Build history of the part. All positions in model axes, mm. Give positions to 0.01 mm unless a question says otherwise; leave off trailing zeros. Loops run counter-clockwise (first coordinate to the right, second up) from the corner with the lowest first, then second, coordinate; pieces in that order, holes last. Notation, with made-up numbers: (0.25, 72) -> (34.25, 72) arc R33 ccw to (34.25, 105) -> close; hole circle Ø2 at (49.25, 57). An arc over 180 degrees is marked (long way). Answer as a JSON object with one key per item and string values. Group by question number.
Q1. Band-saw the part on D-D, the plane x = 14.5. Write the cut outline in (y, z).
Q2. Wall check: probe 1 along Z at (x, y) = (1.5, 0.1); probe 2 along Z at (x, y) = (1, 0.8); probe 3 along X at (y, z) = (0.35, -5.9). Give the ranges that are in metal, low to high. Write a range as from..to.
Q3. Band-saw the part on B-B, the plane x = 1.6. Write the cut outline in (y, z), plus the area to 3 significant figures.
Q4. Band-saw the part on C-C, the plane y = 0.2. Write the cut outline in (x, z), plus the area to 3 significant figures.
Q5. Band-saw the part on A-A, the plane z = 5.9. Write the cut outline in (x, y), plus the area to 3 significant figures.
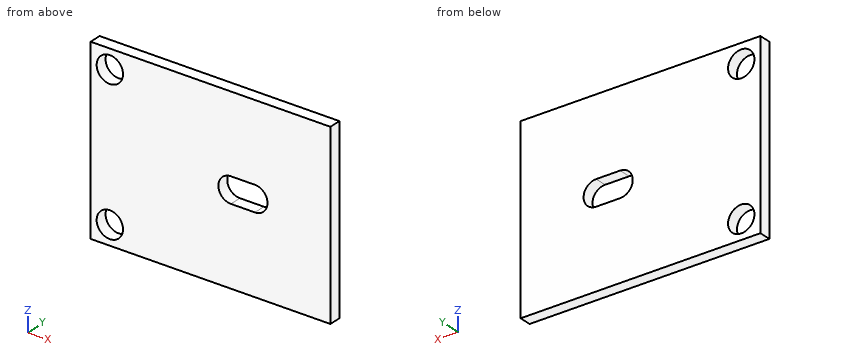
from build123d import *

# Parameters (mm, degrees)
ESQUISSE1_W             = 20
ESQUISSE1_H             = 15
BOSS_EXTRU_1_DEPTH      = 1
ESQUISSE2_R             = 1.1
ENL_V_MAT_EXTRU_1_DEPTH = 22.38340478


with BuildPart() as part:
    # Esquisse1 → Boss.-Extru.1 (new body)
    with BuildSketch(Plane(origin=(0, 0, 0), x_dir=(1, 0, 0), z_dir=(0, 1, 0))):
        with Locations((10, 0)):
            Rectangle(ESQUISSE1_W, ESQUISSE1_H)
    extrude(amount=BOSS_EXTRU_1_DEPTH)

    # Esquisse2 → Enlèv. mat.-Extru.1 (cut, through all)
    with BuildSketch(Plane(origin=(0, 1, 0), x_dir=(1, 0, 0), z_dir=(0, 1, 0))):
        with Locations(Location((1.6, 5.9, 0), (0, 0, 270))):
            Circle(ESQUISSE2_R)
        with Locations(Location((1.6, -5.9, 0), (0, 0, 270))):
            Circle(ESQUISSE2_R)
        with BuildLine():
            Line((11.7, 1.05), (13.7, 1.05))
            ThreePointArc((13.7, 1.05), (14.75, 0), (13.7, -1.05))
            Line((13.7, -1.05), (11.7, -1.05))
            ThreePointArc((11.7, -1.05), (10.65, 0), (11.7, 1.05))
        make_face()
    extrude(amount=-ENL_V_MAT_EXTRU_1_DEPTH, mode=Mode.SUBTRACT)


solid = part.part
Worked answers:
{
 "1": {"outline": "(0, -7.5) -> (1, -7.5) -> (1, -0.68) -> (0, -0.68) -> close; (0, 0.68) -> (1, 0.68) -> (1, 7.5) -> (0, 7.5) -> close"},
 "2": {"probe 1": "-7.5..-7, -4.8..4.8, 7..7.5", "probe 2": "-7.5..-6.82, -4.98..4.98, 6.82..7.5", "probe 3": "0..0.5, 2.7..20"},
 "3": {"outline": "(0, -7.5) -> (1, -7.5) -> (1, -7) -> (0, -7) -> close; (0, -4.8) -> (1, -4.8) -> (1, 4.8) -> (0, 4.8) -> close; (0, 7) -> (1, 7) -> (1, 7.5) -> (0, 7.5) -> close", "area": "10.6 mm2"},
 "4": {"outline": "(0, -7.5) -> (20, -7.5) -> (20, 7.5) -> (0, 7.5) -> close; hole circle Ø2.2 at (1.6, -5.9); hole circle Ø2.2 at (1.6, 5.9); hole (11.7, -1.05) -> (13.7, -1.05) arc R1.05 ccw to (13.7, 1.05) -> (11.7, 1.05) arc R1.05 ccw to start", "area": "285 mm2"},
 "5": {"outline": "(0, 0) -> (0.5, 0) -> (0.5, 1) -> (0, 1) -> close; (2.7, 0) -> (20, 0) -> (20, 1) -> (2.7, 1) -> close", "area": "17.8 mm2"}
}
